Input: part model. Units: mm. Frame: model coordinates. A direction names the side the tool comes from. Coordinates: 2 decimals unless noted, no trailing zeros. Write each loop counter-clockwise with the first axis right and the second up, starting at its lowest first coordinate (ties: lowest second). Pieces come first, ordered by that corner, then holes.
from build123d import *

# Parameters (mm, degrees)
F0_W     = 1
F0_H     = 1
F0_H_2   = 4
F0_W_2   = 4
F0_H_3   = 3
F0_W_3   = 3
F1_DEPTH = 5


with BuildPart() as f1:
    # F0 (on Top) → F1 (new body)
    with BuildSketch(Plane.XY):
        Polygon((0, 20), (0, 0), (5, 0), (5, 1), (1, 1), (1, 4), (1, 5), (1, 9), (1, 10), (1, 14), (1, 15), (1, 19), (4, 19), (4, 15), (4, 14), (5, 14), (5, 15), (5, 20), align=None)
        with Locations((5.5, 14.5)):
            Rectangle(F0_W, F0_H)
        Polygon((10, 15), (6, 15), (6, 14), (9, 14), (9, 10), (9, 9), (10, 9), (10, 10), align=None)
        with Locations((10.5, 9.5)):
            Rectangle(F0_W, F0_H)
        Polygon((15, 10), (11, 10), (11, 9), (14, 9), (14, 5), (14, 4), (15, 4), (15, 5), align=None)
        with Locations((10.5, 7)):
            Rectangle(F0_W, F0_H_2)
        with Locations((5.5, 9.5)):
            Rectangle(F0_W, F0_H)
        with Locations((5.5, 12)):
            Rectangle(F0_W, F0_H_2)
        with Locations((3, 9.5)):
            Rectangle(F0_W_2, F0_H)
        with Locations((5.5, 7)):
            Rectangle(F0_W, F0_H_2)
        with Locations((3, 4.5)):
            Rectangle(F0_W_2, F0_H)
        with Locations((5.5, 2.5)):
            Rectangle(F0_W, F0_H_3)
        with Locations((5.5, 4.5)):
            Rectangle(F0_W, F0_H)
        with Locations((5.5, 0.5)):
            Rectangle(F0_W, F0_H)
        with Locations((8, 0.5)):
            Rectangle(F0_W_2, F0_H)
        with Locations((8, 4.5)):
            Rectangle(F0_W_2, F0_H)
        with Locations((10.5, 4.5)):
            Rectangle(F0_W, F0_H)
        with Locations((10.5, 2.5)):
            Rectangle(F0_W, F0_H_3)
        with Locations((10.5, 0.5)):
            Rectangle(F0_W, F0_H)
        with Locations((13, 0.5)):
            Rectangle(F0_W_2, F0_H)
        with Locations((12.5, 4.5)):
            Rectangle(F0_W_3, F0_H)
        with Locations((15.5, 4.5)):
            Rectangle(F0_W, F0_H)
        with Locations((15.5, 2.5)):
            Rectangle(F0_W, F0_H_3)
        with Locations((15.5, 0.5)):
            Rectangle(F0_W, F0_H)
        Polygon((16, 1), (16, 0), (20, 0), (20, 5), (16, 5), (16, 4), (19, 4), (19, 1), align=None)
        with Locations((7.5, 9.5)):
            Rectangle(F0_W_3, F0_H)
        with Locations((2.5, 14.5)):
            Rectangle(F0_W_3, F0_H)
    extrude(amount=F1_DEPTH)


solid = f1.part
Item 1: Access query for faces 1 (the face through (13, 10, 2)), 2 (the face through (6, 7, 2)), 3 (the face through (20, 2, 2)). Directions: +Z, -Z, +X, -X, +Y, -Y. A direction counts if a zero-diameter tool reaches every point of the face in a straight line with its end or side. Return the directions, or none.
Item 2: Section query D-D, the plane y = 5.75. Return loops of the section in (x, z).
Item 3: Section query C-C, the plane x = 9.75. Return loops of the section in (y, z).
Item 4: Pin query (flat end, axial travel): pin 1 Ø1 at (x, z) = (11, 4) entering from +Y; pin 2 Ø3 at (y, z) = (7, 2.5) entering from +X; pin 3 Ø3 at (x, z) = (10, 1) entering from +Y; pin 4 Ø1.5 at (x, y) = (2.5, 13) entering from +Z. Return the tip coordinate at first contact, or that it passes through.
Item 5: Section query B-B, the plane y = 18. Return loops of the section in (x, z), then the cut area to 4 significant figures.
Item 6: Pull-direction query (Y, two-part tool) for faces 4 (the face through (3, 1, 2)), 5 (the face through (8.5, 9.3, 5)), 6 (the face through (3, 20, 2)); classes: released by +Y, released by -Y, zero draft, split by the parting line, or undercut.
Item 7: Material intervals for line 1 (X direction, y = 7.75, z = 0.9); line 2 (Y direction, x = 11.25, z = 2.1); line 3 (Y direction, x = 9.5, z = 4.55), sorted ascending.
Item 8: Section query A-A, the plane x = 2. Return loops of the section in (y, z), then the cut area to 3 significant figures.
The answers:
1. face 1: +Z, -Z, +X, +Y
1. face 2: +Z, -Z
1. face 3: +Z, -Z, +X, +Y, -Y
2. outline: (0, 0) - (1, 0) - (1, 5) - (0, 5) - close; (5, 0) - (6, 0) - (6, 5) - (5, 5) - close; (10, 0) - (11, 0) - (11, 5) - (10, 5) - close; (14, 0) - (15, 0) - (15, 5) - (14, 5) - close
3. outline: (0, 0) - (1, 0) - (1, 5) - (0, 5) - close; (4, 0) - (5, 0) - (5, 5) - (4, 5) - close; (9, 0) - (15, 0) - (15, 5) - (9, 5) - close
4. pin 1: stops at y = 10
4. pin 2: stops at x = 15
4. pin 3: stops at y = 15
4. pin 4: passes through
5. outline: (0, 0) - (1, 0) - (1, 5) - (0, 5) - close; (4, 0) - (5, 0) - (5, 5) - (4, 5) - close
5. area: 10.00 mm2
6. face 4: undercut
6. face 5: zero draft
6. face 6: released by +Y
7. line 1: x = 0 to 1, 5 to 6, 10 to 11, 14 to 15
7. line 2: y = 0 to 1, 4 to 5, 9 to 10
7. line 3: y = 0 to 1, 4 to 5, 9 to 15
8. outline: (0, 0) - (1, 0) - (1, 5) - (0, 5) - close; (4, 0) - (5, 0) - (5, 5) - (4, 5) - close; (9, 0) - (10, 0) - (10, 5) - (9, 5) - close; (14, 0) - (15, 0) - (15, 5) - (14, 5) - close; (19, 0) - (20, 0) - (20, 5) - (19, 5) - close
8. area: 25.0 mm2
